from build123d import *

# Parameters (mm, degrees)
SKETCH1_W           = 42.25
SKETCH1_H           = 42.25
BOSS_EXTRUDE1_DEPTH = 54
SKETCH2_R           = 1.5
CUT_EXTRUDE1_DEPTH  = 3
CHAMFER1_SIZE       = 3


with BuildPart() as part:
    # Sketch1 → Boss-Extrude1 (new body)
    with BuildSketch(Plane(origin=(0, 0, 0), x_dir=(1, 0, 0), z_dir=(0, 1, 0))):
        with Locations((21.125, 21.125)):
            Rectangle(SKETCH1_W, SKETCH1_H)
    extrude(amount=BOSS_EXTRUDE1_DEPTH)

    # Sketch2 → Cut-Extrude1 (cut)
    with BuildSketch(Plane(origin=(0, 54, 0), x_dir=(1, 0, 0), z_dir=(0, 1, 0))):
        with Locations(Location((36.625, 36.625, 0), (0, 0, 270))):
            Circle(SKETCH2_R)
        with Locations(Location((5.625, 5.625, 0), (0, 0, 270))):
            Circle(SKETCH2_R)
    extrude(amount=-CUT_EXTRUDE1_DEPTH, mode=Mode.SUBTRACT)

    # Chamfer1
    chamfer1_edges = [part.edges().sort_by_distance(p)[0] for p in [
        (0, 27, -42.25),
        (42.25, 27, -42.25),
        (42.25, 27, 0),
        (0, 27, 0),
    ]]
    chamfer(chamfer1_edges, length=CHAMFER1_SIZE)

    # Sketch3 → Revolve1 (revolve)
    with BuildSketch(Plane.ZY.offset(-21.125)):
        Polygon((-21.125, 54), (-21.125, 333.4), (-25.125, 333.4), (-25.125, 79.4), (-28.075, 79.4), (-28.075, 54), align=None)
    revolve(axis=Axis((21.125, 54, -21.125), (0, 1, 0)))


solid = part.part
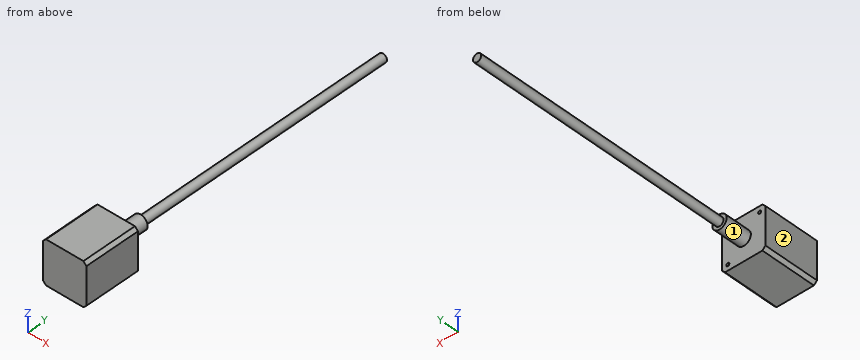
Read the model definition and answer for the solid it produces. Units are mm, in the model's axes. Face numbers are marked on the shaded views. A direction names the side the tool comes from. Give positions to 0.01 mm unless a question says otherwise; leave off trailing zeros. Loops run counter-clockwise (first coordinate to the right, second up) from the corner with the lowest first, then second, coordinate; pieces in that order, holes last. Notation, with made-up numbers: (11, -12) -> (25, -12) arc R11 ccw to (25, 7) -> close; hole circle Ø10 at (6.25, 71). An arc over 180 degrees is marked (long way). Answer as CSV lines item,"result".
Item 1: Each of these flat-tipped pins is pushed along its axis until it touches: pin 1 (12 mm diameter, centred on x = 32, z = -5, fed in from +Y); pin 2 (4 mm diameter, centred on y = 159, z = -19.5, fed in from +X) (3 decimals). Where does it stop, or does it pass through?
Returned:
pin 1,"stops at y = 54"
pin 2,"stops at x = 25.125"
Item 2: Find section C-C on y = 71. Give the vertices of the cut face in (x, z) (3 decimals).
Returned:
outline,"circle Ø13.9 at (21.125, -21.125)"
Item 3: Find section B-B on y = 193. Give the vertices of the cut face in (x, z) (3 decimals), plus the area to 3 significant figures.
Returned:
outline,"circle Ø8 at (21.125, -21.125)"
area,"50.3 mm²"
Item 4: For the marked faces 1 and 2, determine the directions among +Z, -Z, +X, -X, +Y, -Y from which every point of the face is accessible in a straight line to the end or side of a thin tool.
Returned:
face 1,"+Y"
face 2,"+Z, -Z, -X, +Y, -Y"
Item 5: Consider line 1 (Y direction, x = 7, z = -37.5); line 2 (X direction, y = 239.5, z = -21.5); line 3 (Y direction, x = 21, z = -15.5). Determine where each line is inside the solid, lowest interval first. Write a range as [from, to].
Returned:
line 1,"y = [0, 54]"
line 2,"x = [17.14, 25.11]"
line 3,"y = [0, 79.4]"
Item 6: Find section A-A on z = -21.5. Give the vertices of the cut face in (x, y), plus the area to 3 significant figures.
Returned:
outline,"(0, 0) -> (42.25, 0) -> (42.25, 54) -> (28.06, 54) -> (28.06, 79.4) -> (25.11, 79.4) -> (25.11, 333.4) -> (17.14, 333.4) -> (17.14, 79.4) -> (14.19, 79.4) -> (14.19, 54) -> (0, 54) -> close"
area,"4,660 mm²"
